```python
from build123d import *

# Parameters (mm, degrees)
SALIENTE_EXTRUIR1_DEPTH = 7.8
MATRIZL1_DEPTH          = 7.8
CROQUIS2_W              = 7.8
CROQUIS2_H              = 4.999
SALIENTE_EXTRUIR2_DEPTH = 0.801
CROQUIS4_W              = 7.4
CROQUIS4_H              = 7.8
CROQUIS4_R              = 3.1
SALIENTE_EXTRUIR3_DEPTH = 7.87
SALIENTE_EXTRUIR4_START = 0.85
CROQUIS4_3_R            = 3.1
CROQUIS4_3_R_2          = 2.5
SALIENTE_EXTRUIR4_DEPTH = 6.17
REDONDEO2_R             = 3.9


with BuildPart() as part:
    # Croquis1 → Saliente-Extruir1 (new body)
    with BuildSketch(Plane.XY):
        Polygon((0, 0), (3.199966839, 0), (3.199966839, 4.999), (2.398966839, 4.999), (1.598983419, 6.999), (0.799983419, 6.999), (0, 4.999), align=None)
    extrude(amount=SALIENTE_EXTRUIR1_DEPTH)

    # MatrizL1: read off the stored shape, not the designer's step
    # MatrizL1 outline → MatrizL1 (add)
    with BuildSketch(Plane.XY):
        Polygon((0.799983419, 6.999), (0, 4.999), (0, 0), (76.799966839, 0), (76.799966839, 4.999), (75.998966839, 4.999), (75.198983419, 6.999), (74.399983419, 6.999), (73.6, 4.999), (72.798966839, 4.999), (71.998983419, 6.999), (71.199983419, 6.999), (70.4, 4.999), (69.598966839, 4.999), (68.798983419, 6.999), (67.999983419, 6.999), (67.2, 4.999), (66.398966839, 4.999), (65.598983419, 6.999), (64.799983419, 6.999), (64, 4.999), (63.198966839, 4.999), (62.398983419, 6.999), (61.599983419, 6.999), (60.8, 4.999), (59.998966839, 4.999), (59.198983419, 6.999), (58.399983419, 6.999), (57.6, 4.999), (56.798966839, 4.999), (55.998983419, 6.999), (55.199983419, 6.999), (54.4, 4.999), (53.598966839, 4.999), (52.798983419, 6.999), (51.999983419, 6.999), (51.2, 4.999), (50.398966839, 4.999), (49.598983419, 6.999), (48.799983419, 6.999), (48, 4.999), (47.198966839, 4.999), (46.398983419, 6.999), (45.599983419, 6.999), (44.8, 4.999), (43.998966839, 4.999), (43.198983419, 6.999), (42.399983419, 6.999), (41.6, 4.999), (40.798966839, 4.999), (39.998983419, 6.999), (39.199983419, 6.999), (38.4, 4.999), (37.598966839, 4.999), (36.798983419, 6.999), (35.999983419, 6.999), (35.2, 4.999), (34.398966839, 4.999), (33.598983419, 6.999), (32.799983419, 6.999), (32, 4.999), (31.198966839, 4.999), (30.398983419, 6.999), (29.599983419, 6.999), (28.8, 4.999), (27.998966839, 4.999), (27.198983419, 6.999), (26.399983419, 6.999), (25.6, 4.999), (24.798966839, 4.999), (23.998983419, 6.999), (23.199983419, 6.999), (22.4, 4.999), (21.598966839, 4.999), (20.798983419, 6.999), (19.999983419, 6.999), (19.2, 4.999), (18.398966839, 4.999), (17.598983419, 6.999), (16.799983419, 6.999), (16, 4.999), (15.198966839, 4.999), (14.398983419, 6.999), (13.599983419, 6.999), (12.8, 4.999), (11.998966839, 4.999), (11.198983419, 6.999), (10.399983419, 6.999), (9.6, 4.999), (8.798966839, 4.999), (7.998983419, 6.999), (7.199983419, 6.999), (6.4, 4.999), (5.598966839, 4.999), (4.798983419, 6.999), (3.999983419, 6.999), (3.2, 4.999), (2.398966839, 4.999), (1.598983419, 6.999), align=None)
    extrude(amount=MATRIZL1_DEPTH)

    # Croquis2 → Saliente-Extruir2 (add)
    with BuildSketch(Plane.ZY):
        with Locations((3.9, 2.4995)):
            Rectangle(CROQUIS2_W, CROQUIS2_H)
    extrude(amount=SALIENTE_EXTRUIR2_DEPTH)

    # Croquis4 → Saliente-Extruir3 (add)
    # profile 1 of 2: a face of its own
    with BuildSketch(Plane(origin=(0, 0, 0), x_dir=(1, 0, 0), z_dir=(0, 1, 0))):
        with Locations((-4.501, -3.9)):
            Rectangle(CROQUIS4_W, CROQUIS4_H)
        with Locations(Location((-4.501, -3.9, 0), (0, 0, 270))):
            Circle(CROQUIS4_R, mode=Mode.SUBTRACT)
    # profile 2 of 2: a face of its own
    with BuildSketch(Plane(origin=(0, 0, 0), x_dir=(1, 0, 0), z_dir=(0, 1, 0))):
        with Locations((80.499966839, -3.9)):
            Rectangle(CROQUIS4_W, CROQUIS4_H)
        with Locations(Location((80.499966839, -3.9, 0), (0, 0, 270))):
            Circle(CROQUIS4_R, mode=Mode.SUBTRACT)
    extrude(amount=SALIENTE_EXTRUIR3_DEPTH)

    # Croquis4<3> → Saliente-Extruir4 (add)
    # profile 1 of 2: a face of its own
    with BuildSketch(Plane(origin=(0, 0, 0), x_dir=(1, 0, 0), z_dir=(0, 1, 0)).offset(SALIENTE_EXTRUIR4_START)):
        with Locations(Location((-4.501, -3.9, 0), (0, 0, 270))):
            Circle(CROQUIS4_3_R)
        with Locations(Location((-4.501, -3.9, 0), (0, 0, 270))):
            Circle(CROQUIS4_3_R_2, mode=Mode.SUBTRACT)
    # profile 2 of 2: a face of its own
    with BuildSketch(Plane(origin=(0, 0, 0), x_dir=(1, 0, 0), z_dir=(0, 1, 0)).offset(SALIENTE_EXTRUIR4_START)):
        with Locations(Location((80.499966839, -3.9, 0), (0, 0, 270))):
            Circle(CROQUIS4_3_R)
        with Locations(Location((80.499966839, -3.9, 0), (0, 0, 270))):
            Circle(CROQUIS4_3_R_2, mode=Mode.SUBTRACT)
    extrude(amount=SALIENTE_EXTRUIR4_DEPTH)

    # Redondeo2
    redondeo2_edges = [part.edges().sort_by_distance(p)[0] for p in [
        (84.199966839, 3.935, 0),
        (84.199966839, 3.935, 7.8),
        (-8.201, 3.935, 0),
        (-8.201, 3.935, 7.8),
    ]]
    fillet(redondeo2_edges, radius=REDONDEO2_R - 0.0001)  # a hair under: the kernel refuses the full size


solid = part.part
```
The model under review builds one solid part; all positions refer to its coordinate system, in mm. A direction names the side the tool comes from. Round coordinates to 2 decimals unless told otherwise and drop trailing zeros. Use a Markdown table: item, result.
1) Draft analysis for pull direction Z (two halves, no side actions). For faces 1 (the face through (37, 3, 0)), 2 (the face through (61.2, 6, 3.8)), 3 (the face through (83.574, 7.439, 3.496)), state which applies: released by +Z, released by -Z, zero draft, split by the parting line, or undercut.
Report:
| item | result |
|---|---|
| face 1 | released by -Z |
| face 2 | zero draft |
| face 3 | undercut |
2) Insertion check: pin 1 (0.9 mm diameter, centred on x = 71.5, z = 5.5, fed in from +Y); pin 2 (2 mm diameter, centred on y = 3, z = 2.5, fed in from +X); pin 3 (3 mm diameter, centred on y = 7, z = 7, fed in from -X). Each pin has a flat end and moves straight along its axis. Give the tip position at first contact, or say it passes through.
Report:
| item | result |
|---|---|
| pin 1 | y = 7 |
| pin 2 | x = 84.18 |
| pin 3 | x = -7.86 |
3) Consider section A-A (y = 5.75). Give the number of separate pieces and of enclosed holes in the cut face, then the cut area to 3 significant figures.
Report:
| item | result |
|---|---|
| separate pieces | 26 |
| enclosed holes | 2 |
| area | 400 mm^2 |
4) Wall thickness on line 1 along X through (y, z) = (3, 4); line 2 along X through (y, z) = (3.25, 5.75); line 3 along Z through (x, y) = (80.5, 4): over which ranges is each line inside the solid? List them lowest first. Write a range as [from, to].
Report:
| item | result |
|---|---|
| line 1 | [-8.2, -7], [-2, 78], [83, 84.2] |
| line 2 | [-7.73, -6.18], [-2.82, 78.82], [82.18, 83.73] |
| line 3 | [0.01, 1.4], [6.4, 7.79] |
5) Tool access review of faces 4 (the face through (-4, 0.85, 1)), 5 (the face through (77, 7.87, 4)), 6 (the face through (32.4, 6, 3.8)): name each direction out of +Z, -Z, +X, -X, +Y, -Y from which nothing blocks a thin tool from reaching the whole face with its end or side.
Report:
| item | result |
|---|---|
| face 4 | -Y |
| face 5 | +Z, -Z, +X, -X, +Y |
| face 6 | +Z, -Z, +Y |
